Input: part model. Units: mm. Frame: model coordinates. Give positions to 0.01 mm unless a question says otherwise; leave off trailing zeros. Loops run counter-clockwise (first coordinate to the right, second up) from the corner with the lowest first, then second, coordinate; pieces in that order, holes last. Notation, with made-up numbers: (72, 11.25) -> (122, 11.25) arc R20 ccw to (122, 29.25) -> close; hole circle Ø5 at (88, 26). An arc over 180 degrees is marked (long way). One line per question, with ' | ' between items.
from build123d import *

# Parameters (mm, degrees)
CROQUIS1_R              = 70
CROQUIS1_R_2            = 4.5
SALIENTE_EXTRUIR1_DEPTH = 3


with BuildPart() as part:
    # Croquis1 → Saliente-Extruir1 (new body)
    with BuildSketch(Plane(origin=(0, 0, 0), x_dir=(1, 0, 0), z_dir=(0, 1, 0))):
        with Locations(Location((0, 0, 0), (0, 0, 270))):
            Circle(CROQUIS1_R)
        with Locations(Location((0, 0, 0), (0, 0, 270))):
            Circle(CROQUIS1_R_2, mode=Mode.SUBTRACT)
        Polygon((0, 11), (7, 11), (7, 14), (14.5, 14), (14.5, 31), (-14.5, 31), (-14.5, 14), (-7, 14), (-7, 11), align=None, mode=Mode.SUBTRACT)
        Polygon((24.748737342, 24.748737342), (31.819805153, 17.67766953), (33.941125497, 19.798989873), (19.798989873, 33.941125497), (17.67766953, 31.819805153), align=None, mode=Mode.SUBTRACT)
        Polygon((11, 0), (11, 7), (14, 7), (14, 9), (17, 9), (17, 0), (17, -9), (14, -9), (14, -7), (11, -7), align=None, mode=Mode.SUBTRACT)
        Polygon((-24.748737342, 24.748737342), (-17.67766953, 31.819805153), (-19.798989873, 33.941125497), (-33.941125497, 19.798989873), (-31.819805153, 17.67766953), align=None, mode=Mode.SUBTRACT)
        Polygon((-14, -7), (-11, -7), (-11, 0), (-11, 7), (-14, 7), (-14, 9), (-17, 9), (-17, -9), (-14, -9), align=None, mode=Mode.SUBTRACT)
        Polygon((-7, -14), (-9, -14), (-9, -17), (0, -17), (9, -17), (9, -14), (7, -14), (7, -11), (0, -11), (-7, -11), align=None, mode=Mode.SUBTRACT)
        Polygon((24.748737342, -24.748737342), (17.67766953, -31.819805153), (19.798989873, -33.941125497), (33.941125497, -19.798989873), (31.819805153, -17.67766953), align=None, mode=Mode.SUBTRACT)
        Polygon((-24.748737342, -24.748737342), (-31.819805153, -17.67766953), (-33.941125497, -19.798989873), (-19.798989873, -33.941125497), (-17.67766953, -31.819805153), align=None, mode=Mode.SUBTRACT)
        Polygon((0, 62), (20, 62), (20, 59), (-20, 59), (-20, 62), align=None, mode=Mode.SUBTRACT)
        Polygon((55.861435714, 27.577164466), (27.577164466, 55.861435714), (29.69848481, 57.982756057), (43.840620434, 43.840620434), (57.982756057, 29.69848481), align=None, mode=Mode.SUBTRACT)
        Polygon((59, -20), (59, 20), (62, 20), (62, 0), (62, -20), align=None, mode=Mode.SUBTRACT)
        Polygon((27.577164466, -55.861435714), (55.861435714, -27.577164466), (57.982756057, -29.69848481), (43.840620434, -43.840620434), (29.69848481, -57.982756057), align=None, mode=Mode.SUBTRACT)
        Polygon((-20, -59), (20, -59), (20, -62), (0, -62), (-20, -62), align=None, mode=Mode.SUBTRACT)
        Polygon((-55.861435714, -27.577164466), (-27.577164466, -55.861435714), (-29.69848481, -57.982756057), (-43.840620434, -43.840620434), (-57.982756057, -29.69848481), align=None, mode=Mode.SUBTRACT)
        Polygon((-59, 20), (-59, -20), (-62, -20), (-62, 0), (-62, 20), align=None, mode=Mode.SUBTRACT)
        Polygon((-27.577164466, 55.861435714), (-55.861435714, 27.577164466), (-57.982756057, 29.69848481), (-43.840620434, 43.840620434), (-29.69848481, 57.982756057), align=None, mode=Mode.SUBTRACT)
    extrude(amount=SALIENTE_EXTRUIR1_DEPTH)


solid = part.part
1. Section query B-B (x = 0). Output: boundary loops of the cut face in (y, z).
Determined:
outline: (0, -70) -> (3, -70) -> (3, -62) -> (0, -62) -> close; (0, -59) -> (3, -59) -> (3, -31) -> (0, -31) -> close; (0, -11) -> (3, -11) -> (3, -4.5) -> (0, -4.5) -> close; (0, 4.5) -> (3, 4.5) -> (3, 11) -> (0, 11) -> close; (0, 17) -> (3, 17) -> (3, 59) -> (0, 59) -> close; (0, 62) -> (3, 62) -> (3, 70) -> (0, 70) -> close
2. Pin query (flat end, axial travel): P1, Ø1.5, axis at x = -4, y = 2, coming from the +Z side; P2, Ø1, axis at y = 2, z = 8.5, coming from the +X side; P3, Ø1.5, axis at y = 1.5, z = -12, coming from the +X side. Return the tip coordinate at first contact, or that it passes through.
Determined:
P1: stops at z = 69.92 | P2: stops at x = 69.54 | P3: stops at x = 69.09
3. Section query A-A (z = 0). Output: boundary loops of the cut face in (x, y), then the cut area to 3 significant figures.
Determined:
outline: (-70, 0) -> (-62, 0) -> (-62, 3) -> (-70, 3) -> close; (-59, 0) -> (-17, 0) -> (-17, 3) -> (-59, 3) -> close; (-11, 0) -> (-4.5, 0) -> (-4.5, 3) -> (-11, 3) -> close; (4.5, 0) -> (11, 0) -> (11, 3) -> (4.5, 3) -> close; (17, 0) -> (59, 0) -> (59, 3) -> (17, 3) -> close; (62, 0) -> (70, 0) -> (70, 3) -> (62, 3) -> close | area: 339 mm2
4. Ray query, line 1 along X through (y, z) = (0.7, 0); line 2 along X through (y, z) = (1.15, 31.5); line 3 along Z through (x, y) = (-44.5, 2). Return the intervals inside material, ascending. Write a range as from..to.
Determined:
line 1: x = -70..-62, -59..-17, -11..-4.5, 4.5..11, 17..59, 62..70 | line 2: x = -62.51..-56.18, -51.94..-22.24, -18..18, 22.24..51.94, 56.18..62.51 | line 3: z = -54.03..-43.18, -38.94..38.94, 43.18..54.03
5. Section query D-D (y = 0.85). Count the separate pieces of the cut face and the enclosed holes in it, then the cut area to 3 significant figures.
Determined:
separate pieces: 1 | enclosed holes: 17 | area: 13,300 mm2
6. Section query C-C (z = 51.5). Output: boundary loops of the cut face in (x, y), then the cut area to 3 significant figures.
Determined:
outline: (-47.41, 0) -> (-36.18, 0) -> (-36.18, 3) -> (-47.41, 3) -> close; (-31.94, 0) -> (31.94, 0) -> (31.94, 3) -> (-31.94, 3) -> close; (36.18, 0) -> (47.41, 0) -> (47.41, 3) -> (36.18, 3) -> close | area: 259 mm2
7. Pull-direction query (Z, two-part tool) for faces 1 (the cylindrical face through (-42.594, 1.479, -55.55)), 2 (the flat face through (0, 1, -31)), 3 (the flat face through (14.5, 1, -22)), 4 (the flat face through (17, 0, -17)); classes: pulls with the +Z half, pulls with the -Z half, needs draft (parallel to the pull), parting line crosses it, or undercut.
Determined:
face 1: parting line crosses it | face 2: undercut | face 3: undercut | face 4: needs draft
